Build history of the part. All positions in model axes, mm. A direction names the side the tool comes from. Give positions to 0.01 mm unless a question says otherwise; leave off trailing zeros. Loops run counter-clockwise (first coordinate to the right, second up) from the corner with the lowest first, then second, coordinate; pieces in that order, holes last. Notation, with made-up numbers: (52.25, 28) -> (109.25, 28) arc R17 cw to (109.25, 33) -> close; hole circle Ø2 at (31, 21.25). An arc over 180 degrees is marked (long way). One line per question, with ' | ' between items. Start each with the question number.
(1) Mould opens along X. For faces 3 (the face through (-0.43, -82.04, 0.25)), 4 (the face through (60, 37, 0)), 5 (the face through (-56.917, 50.273, 0.258)) say: pulls with the +X half, pulls with the -X half, needs draft (parallel to the pull), parting line crosses it, or undercut.
(2) 3-axis set-ups, long thin cutter, end or side, ignore diameter. For faces 1 (the face through (-4.7, -75.6, 0.3)), 2 (the face through (82.04, -0.43, 0.25)): which of +Z, -Z, +X, -X, +Y, -Y reach the whole face in a straight line?
(3) Drill centre lines: L1, parallel to X at y = -45, z = 0.2; L2, parallel to Y at x = 20, z = 0.15; L3, parallel to X at y = -62.5, z = 0.2. Where is each one in solid material? Low to high. Write a range as from..to.
(4) Slice it at C-C, the plane z = 0.4. Give the number of separate pieces and of enclosed holes in the cut face, then the cut area to 3 significant figures.
(5) Slice it at B-B, the plane y = -19.5. Write the cut outline in (x, z), then the cut area to 3 significant figures.
(6) Slice it at D-D, the plane y = 23. Write the cut outline in (x, z), then the cut area to 3 significant figures.
(7) Slice it at A-A, the plane x = -17.5. Write the cut outline in (y, z).
```python
from build123d import *

# Parameters (mm, degrees)
SKETCH4_R           = 82.042
BOSS_EXTRUDE2_DEPTH = 0.508
SKETCH5_R           = 69.342
CUT_EXTRUDE5_DEPTH  = 1.508
SKETCH6_R           = 4.699
CUT_EXTRUDE6_DEPTH  = 1.508
CUT_EXTRUDE11_DEPTH = 1.508


with BuildPart() as part:
    # Sketch4 → Boss-Extrude2 (new body)
    with BuildSketch(Plane.XY):
        Circle(SKETCH4_R)
    extrude(amount=BOSS_EXTRUDE2_DEPTH)

    # Sketch5 → Cut-Extrude5 (cut, through all)
    with BuildSketch(Plane.XY.offset(0.508)):
        Circle(SKETCH5_R)
    extrude(amount=-CUT_EXTRUDE5_DEPTH, mode=Mode.SUBTRACT)

    # Sketch6 → Cut-Extrude6 (cut, through all)
    with BuildSketch(Plane.XY.offset(0.508)):
        with Locations((75.692, 0)):
            Circle(SKETCH6_R)
        with BuildLine():
            ThreePointArc((56.845020598, -56.845021895), (56.845021284, -50.199631755), (50.199631144, -50.199632289))
            ThreePointArc((50.199631144, -50.199632289), (27.167844051, -65.588980009), (-1.058e-06, -70.993))
            ThreePointArc((-1.058e-06, -70.993), (-4.699, -75.69199993), (-1.198e-06, -80.391))
            ThreePointArc((-1.198e-06, -80.391), (30.764302834, -74.271599903), (56.845020598, -56.845021895))
        make_face()
        with BuildLine():
            ThreePointArc((-56.845021895, -56.845020598), (-50.199631755, -56.845021284), (-50.199632289, -50.199631144))
            ThreePointArc((-50.199632289, -50.199631144), (-65.588980009, -27.167844051), (-70.993, 1.058e-06))
            ThreePointArc((-70.993, 1.058e-06), (-75.69199993, 4.699), (-80.391, 1.198e-06))
            ThreePointArc((-80.391, 1.198e-06), (-74.271599903, -30.764302834), (-56.845021895, -56.845020598))
        make_face()
        with BuildLine():
            ThreePointArc((-56.845020598, 56.845021895), (-56.845021284, 50.199631755), (-50.199631144, 50.199632289))
            ThreePointArc((-50.199631144, 50.199632289), (-27.167844051, 65.588980009), (1.058e-06, 70.993))
            ThreePointArc((1.058e-06, 70.993), (4.699, 75.69199993), (1.198e-06, 80.391))
            ThreePointArc((1.198e-06, 80.391), (-30.764302834, 74.271599903), (-56.845020598, 56.845021895))
        make_face()
    extrude(amount=-CUT_EXTRUDE6_DEPTH, mode=Mode.SUBTRACT)

    # Sketch8 → Cut-Extrude11 (cut, through all)
    with BuildSketch(Plane.XY.offset(0.508)):
        Polygon((76.869596069, 30.465791131), (75.89758015, 32.812445144), (74.724253144, 32.326437185), (75.696269062, 29.979783172), align=None)
        Polygon((-30.465791131, 76.869596069), (-32.812445144, 75.89758015), (-32.326437185, 74.724253144), (-29.979783172, 75.696269062), align=None)
        Polygon((-75.89758015, 32.812445144), (-76.869596069, 30.465791131), (-75.696269062, 29.979783172), (-74.724253144, 32.326437185), align=None)
        Polygon((-76.869596069, -30.465791131), (-75.89758015, -32.812445144), (-74.724253144, -32.326437185), (-75.696269062, -29.979783172), align=None)
        Polygon((-32.812445144, -75.89758015), (-30.465791131, -76.869596069), (-29.979783172, -75.696269062), (-32.326437185, -74.724253144), align=None)
        Polygon((30.465791131, -76.869596069), (32.812445144, -75.89758015), (32.326437185, -74.724253144), (29.979783172, -75.696269062), align=None)
        Polygon((75.89758015, -32.812445144), (76.869596069, -30.465791131), (75.696269062, -29.979783172), (74.724253144, -32.326437185), align=None)
        Polygon((32.812445144, 75.89758015), (30.465791131, 76.869596069), (29.979783172, 75.696269062), (32.326437185, 74.724253144), align=None)
    extrude(amount=-CUT_EXTRUDE11_DEPTH, mode=Mode.SUBTRACT)


solid = part.part
```
Final values:
1) face 3: parting line crosses it | face 4: needs draft | face 5: undercut
2) face 1: +Z, -Z | face 2: +Z, -Z, +X
3) L1: -68.6..-66.62, -54.91..-52.76, 52.76..68.6 | L2: -79.57..-77.86, -68.12..-66.4, 66.4..79.57 | L3: -53.15..-30.03, 30.03..33.67, 50.56..53.15
4) separate pieces: 1 | enclosed holes: 5 | area: 4,070 mm2
5) outline: (-79.69, 0) -> (-77.99, 0) -> (-77.99, 0.51) -> (-79.69, 0.51) -> close; (-68.26, 0) -> (-66.54, 0) -> (-66.54, 0.51) -> (-68.26, 0.51) -> close; (66.54, 0) -> (79.69, 0) -> (79.69, 0.51) -> (66.54, 0.51) -> close | area: 8.42 mm2
6) outline: (-78.75, 0) -> (-65.42, 0) -> (-65.42, 0.51) -> (-78.75, 0.51) -> close; (65.42, 0) -> (78.75, 0) -> (78.75, 0.51) -> (65.42, 0.51) -> close | area: 13.5 mm2
7) outline: (-80.15, 0) -> (-67.1, 0) -> (-67.1, 0.51) -> (-80.15, 0.51) -> close; (67.1, 0) -> (68.8, 0) -> (68.8, 0.51) -> (67.1, 0.51) -> close; (78.46, 0) -> (80.15, 0) -> (80.15, 0.51) -> (78.46, 0.51) -> close
